Autodesk Inventor part; units mm, degrees
ref_plane "YZ Plane" through (0, 0, 0) normal (1, 0, 0) x (0, 1, 0)
ref_plane "XZ Plane" through (0, 0, 0) normal (0, 1, 0) x (-1, 0, 0)
ref_plane "XY Plane" through (0, 0, 0) normal (0, 0, 1) x (1, 0, 0)
sketch "Sketch1" plane through (0, 0, 0) normal (0, 0, 1) x (1, 0, 0)
  line L0 (0, 19.05) -> (0, 0)
  line L1 (0, 19.05) -> (42.2604, 19.05)
  line L2 (42.2604, 19.05) -> (42.2604, 0)
  line L3 (42.2604, 0) -> (0, 0)
  line L4 (0, 19.05) -> (0, 57.15)
  line L5 (0, 57.15) -> (19.05, 57.15)
  line L6 (19.05, 57.15) -> (19.05, 19.05)
  line L7 (0, 38.1) -> (19.05, 38.1)
  dimension "d0" = 19.05
  dimension "d1" = 19.05
  dimension "d2" = 38.1
extrude "Extrusion1" add sketch "Sketch1" against normal blind 19.05
sketch "straight 3 cube" plane through (0, 0, 0) normal (0, 0, 1) x (1, 0, 0)
  line L0 (19.05, 19.05) -> (42.2604, 19.05)
  line L1 (19.05, 19.05) -> (0, 19.05)
  line L2 (0, 0) -> (0, 57.15)
  line L3 (19.05, 19.05) -> (19.05, 38.1)
  line L4 (19.05, 57.15) -> (19.05, 19.05)
  line L5 (19.05, 38.1) -> (0, 38.1)
  line L6 (19.05, 19.05) -> (0, 19.05)
  line L7 (19.05, 19.05) -> (0, 19.05)
  line L8 (19.05, 19.05) -> (19.05, 38.1)
  line L9 (0, 38.1) -> (19.05, 38.1)
  line L10 (19.05, 38.1) -> (0, 38.1)
  line L11 (0, 38.1) -> (0, 19.05)
  line L12 (0, 19.05) -> (19.05, 19.05)
  line L13 (19.05, 19.05) -> (19.05, 38.1)
  line L14 (19.05, 19.05) -> (0, 19.05)
sketch "Sketch3" plane through (0, 0, -19.05) normal (0, 0, -1) x (-1, 0, 0)
  line L0 (-19.05, 19.05) -> (-42.2604, 19.05)
  line L1 (-19.05, 19.05) -> (0, 19.05)
  line L2 (0, 0) -> (0, 57.15)
  line L3 (0, 19.05) -> (0, 57.15)
  line L4 (0, 57.15) -> (-19.05, 57.15)
  line L5 (0, 57.15) -> (-19.05, 57.15)
  line L6 (-19.05, 57.15) -> (-19.05, 19.05)
  line L7 (-19.05, 57.15) -> (-19.05, 19.05)
extrude "Extrusion2" add sketch "Sketch3" along normal blind 19.05
sketch "Sketch4" plane through (19.05, 19.05, 0) normal (1, 0, 0) x (0, 0, -1)
  point P0 (0, -19.05)
sketch "Sketch5" plane through (0, 0, 0) normal (0, 0, 1) x (1, 0, 0)
  point P0 (0, 0)
equation "\"d1\" = cube"
equation "\"d2\" = 2 * cube"
equation "\"d3\" = cube"
equation "\"d5\" = cube"
equation "\"BendRadius\" = Thickness"
equation "\"BendReliefWidth\" = Thickness"
equation "\"BendReliefDepth\" = 0.5 * Thickness"
equation "\"CornerReliefSize\" = 4 * Thickness"
equation "\"MinimumRemnant\" = 2 * Thickness"
equation "\"TransitionRadius\" = BendRadius"
equation "\"JacobiRadiusSize\" = BendRadius"
equation "\"GapSize\" = Thickness"
equation "\"cube\" = 19.05"
properties part number "IED7_Sun_PuzzleCubeOrange"
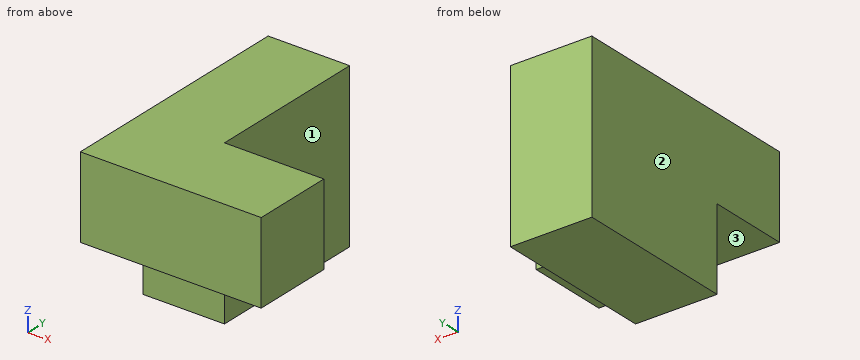
Here's how the part is built. I have some questions about the finished solid (model axes, mm). Face numbers are marked on the shaded views. A direction names the side the tool comes from. Round coordinates to 2 decimals unless told otherwise and drop trailing zeros. Write each loop counter-clockwise with the first axis right and the second up, starting at its lowest first coordinate (ties: lowest second). Pieces come first, ordered by that corner, then holes.
Q1. If we section it at B-B on y = 8.5: Write out the boundary of the cut face in (x, z).
Q2. Please list where these lines run through material, in increasing order: probe 1 along Y at (x, z) = (12.5, -30.5); probe 2 along X at (y, z) = (52, -9.5); probe 3 along Z at (x, y) = (34, 5.5).
Q3. If we section it at A-A on x = 13: Write out the boundary of the cut face in (y, z), plus the area to 3 significant figures.
Q4. If we section it at D-D on z = -32.5: Write out the boundary of the cut face in (x, y).
Q5. Which directions (+Z, -Z, +X, -X, +Y, -Y) give clear straight access to the entire face, cutting with the end or side of a thin tool? Please do the marked faces 1, 2 and 3.
Q6. If we section it at C-C on z = -14.5: Write out the boundary of the cut face in (x, y).
Q7. Will these pins go through, and if not, where does the flat tip stop? P1, Ø9.5, axis at x = 15, y = 8.5, coming from the -Z side; P2, Ø9.5, axis at x = 5.5, z = -25, coming from the -Y side.
Answer below:
1. outline: (0, -19.05) - (42.26, -19.05) - (42.26, 0) - (0, 0) - close
2. probe 1: y = 19.05 to 57.15
2. probe 2: x = 0 to 19.05
2. probe 3: z = -19.05 to 0
3. outline: (0, -19.05) - (19.05, -19.05) - (19.05, -38.1) - (57.15, -38.1) - (57.15, 0) - (0, 0) - close
3. area: 1,810 mm2
4. outline: (0, 19.05) - (19.05, 19.05) - (19.05, 57.15) - (0, 57.15) - close
5. face 1: +Z, -Z, +X, +Y
5. face 2: +Z, -Z, -X, +Y, -Y
5. face 3: -Z, +X, -X, -Y
6. outline: (0, 0) - (42.26, 0) - (42.26, 19.05) - (19.05, 19.05) - (19.05, 57.15) - (0, 57.15) - close
7. P1: stops at z = -19.05
7. P2: stops at y = 19.05
